The figure shows three views and two pictorial views of one solid part (mm, origin at its lowest corner). Answer the questions. A direction names the side the tool comes from. Coordinates: 2 decimals unless noted, no trailing zeros. Loops run counter-clockwise (first coordinate to the right, second up) from the corner with the lowest first, then second, coordinate; pieces in that order, holes last.
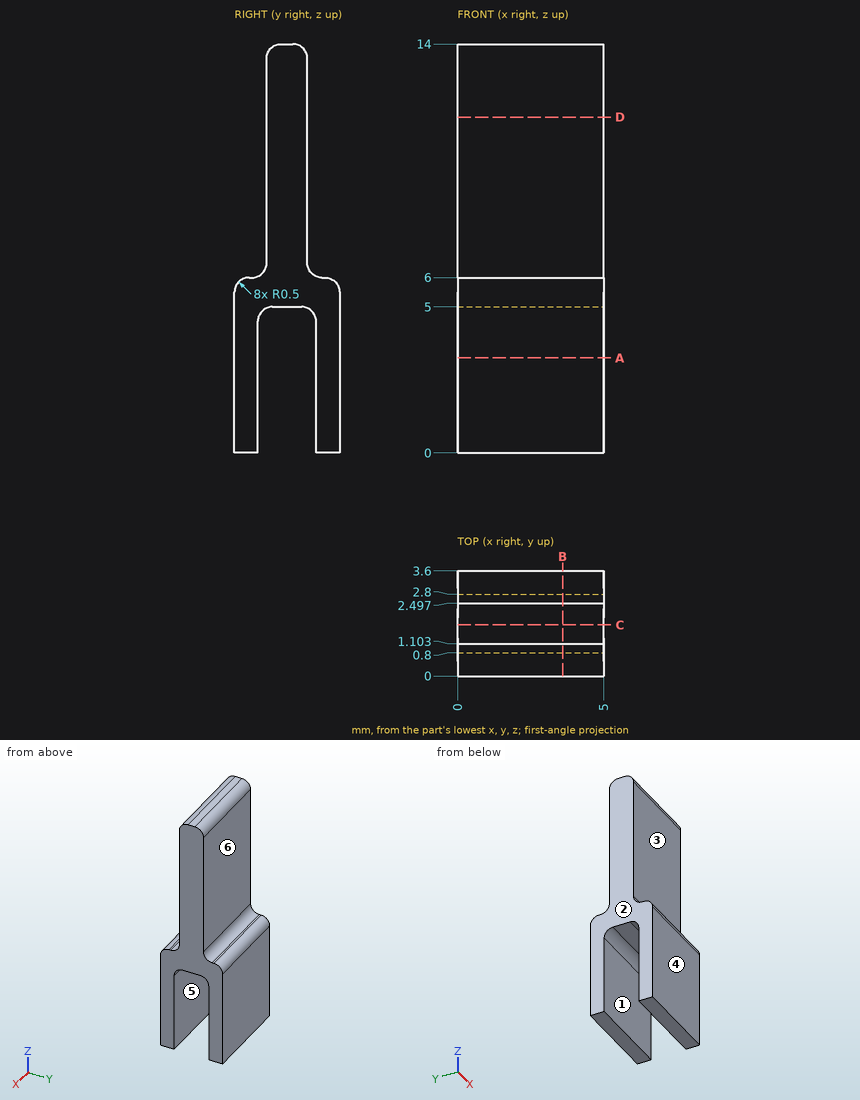
Q1. A cutting plane is placed at B-B (x = 3.6). Give the vertices of the cut face in (y, z).
Findings below:
outline: (0, 0) - (0.8, 0) - (0.8, 4.5) arc R0.5 cw to (1.3, 5) - (2.3, 5) arc R0.5 cw to (2.8, 4.5) - (2.8, 0) - (3.6, 0) - (3.6, 5.5) arc R0.5 ccw to (3.1, 6) - (3, 6) arc R0.5 cw to (2.5, 6.5) - (2.5, 13.5) arc R0.5 ccw to (2, 14) - (1.6, 14) arc R0.5 ccw to (1.1, 13.5) - (1.1, 6.5) arc R0.5 cw to (0.6, 6) - (0.5, 6) arc R0.5 ccw to (0, 5.5) - close
Q2. Straight lines are drawn through the part: probe 1 along Y at (x, z) = (4.05, 0.75); probe 2 along Y at (x, z) = (2.95, 12.75); probe 3 along Z at (x, y) = (1.15, 1.75). For each, find the intervals that lie inside material, in ascending order.
Findings below:
probe 1: y = 0 to 0.8, 2.8 to 3.6
probe 2: y = 1.1 to 2.5
probe 3: z = 5 to 14
Q3. A cutting plane is placed at D-D (z = 11.5). Give the vertices of the cut face in (x, y).
Findings below:
outline: (0, 1.1) - (5, 1.1) - (5, 2.5) - (0, 2.5) - close
Q4. Determine the mould class of the marked faces 4, 5 and 6 for opening direction Y: +Y half, -Y half, draft (parallel to the pull), parting line (faces both ways), or undercut.
Findings below:
face 4: -Y half
face 5: undercut
face 6: +Y half
Q5. A cutting plane is placed at A-A (z = 3.25). Give the vertices of the cut face in (x, y).
Findings below:
outline: (0, 0) - (5, 0) - (5, 0.8) - (0, 0.8) - close; (0, 2.8) - (5, 2.8) - (5, 3.6) - (0, 3.6) - close
Q6. Which of the six approach directions +Z, -Z, +X, -X, +Y, -Y give full straight-line access (tool end or side, diameter ignored) to the marked faces 1, 2 and 3?
Findings below:
face 1: -Z, +X, -X
face 2: +Z, -Z, -X, +Y, -Y
face 3: +Z, +X, -X, -Y
Q7. Flat-ended cylindrical pins translate along their axes: pin 1 Ø1.5 at (x, z) = (2.5, 10) entering from -Y; pin 2 Ø0.5 at (x, y) = (3, 2) entering from -Z. Find the tip coordinate at first contact, or state that the pin passes through.
Findings below:
pin 1: stops at y = 1.1
pin 2: stops at z = 5
Q8. A cutting plane is placed at C-C (y = 1.75). Give the vertices of the cut face in (x, z).
Findings below:
outline: (0, 5) - (5, 5) - (5, 14) - (0, 14) - close
